Print and shaded views of the part. All mm, measured from the part's lowest x, y and z. A direction names the side the tool comes from. Round coordinates to 2 decimals unless told otherwise and drop trailing zeros. Write each loop counter-clockwise with the first axis right and the second up, starting at its lowest first coordinate (ties: lowest second). Pieces come first, ordered by that corner, then holes. Notation, with made-up numbers: (51, -0.5) - (59, -0.5) arc R13 cw to (59, 6.5) - close; hole circle Ø6 at (-21.75, 88.5). An arc over 180 degrees is marked (long way). Put each result on its own line as item: value. Start each with the question number.
Item 1: 3-axis set-ups, long thin cutter, end or side, ignore diameter. For the marked faces 1, 2 and 3: which of +Z, -Z, +X, -X, +Y, -Y reach the whole face in a straight line?
Item 2: Cut at D-D (x = 40.5). Give the cut face in (y, z), and give its area (3 significant figures).
Item 3: Pin check, flat tips, straight feed: pin 1 Ø0.7 at (y, z) = (9.5, 5) entering from -X; pin 2 Ø0.8 at (y, z) = (1.5, 3) entering from -X; pin 3 Ø1.4 at (y, z) = (0.5, 3) entering from +X. Stop position of each tip, or through.
Item 4: Cut at C-C (z = 5). Give the cut face in (x, y), and give its area (3 significant figures).
Item 5: Drill centre lines: line 1 (Y direction, x = 20, z = 4.75); line 2 (X direction, y = 12.75, z = 4.25); line 3 (X direction, y = 10.75, z = 3.5). Where is each one in solid material? Low to high. Write a range as from..to.
Item 6: Cut at A-A (x = 20). Give the cut face in (y, z), and give its area (3 significant figures).
Item 7: Cut at B-B (y = 11.15). Give the cut face in (x, z) (3 decimals), and give its area (3 significant figures).
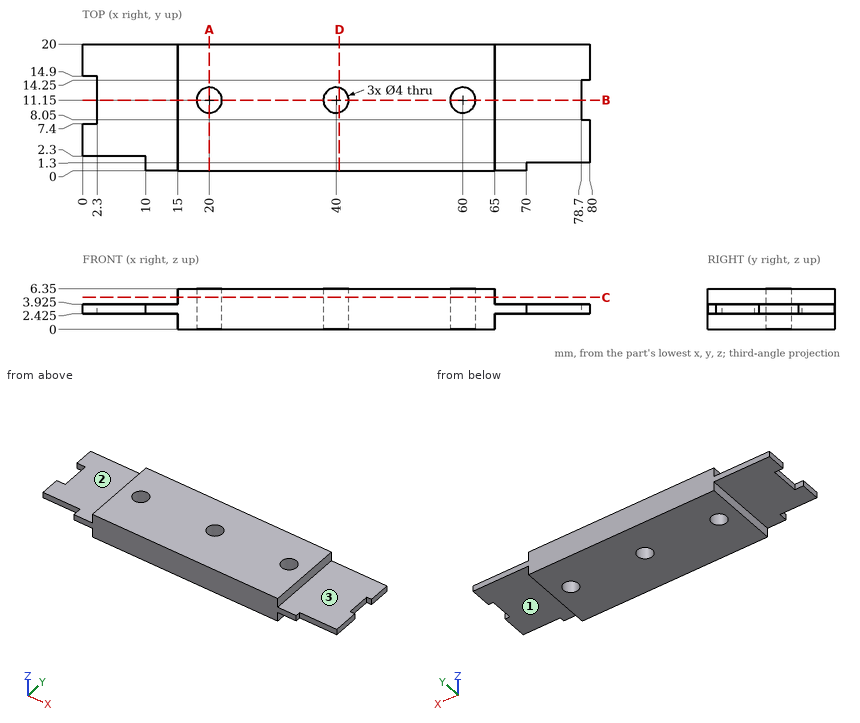
Output values:
1. face 1: -Z, +X, +Y, -Y
1. face 2: +Z, -X, +Y, -Y
1. face 3: +Z, +X, +Y, -Y
2. outline: (0, 0) - (9.21, 0) - (9.21, 6.35) - (0, 6.35) - close; (13.09, 0) - (20, 0) - (20, 6.35) - (13.09, 6.35) - close
2. area: 102 mm2
3. pin 1: x = 15
3. pin 2: x = 10
3. pin 3: x = 70
4. outline: (15, 0) - (65, 0) - (65, 20) - (15, 20) - close; hole circle Ø4 at (20, 11.15); hole circle Ø4 at (40, 11.15); hole circle Ø4 at (60, 11.15)
4. area: 962 mm2
5. line 1: 0..9.15, 13.15..20
5. line 2: 15..18.8, 21.2..38.8, 41.2..58.8, 61.2..65
5. line 3: 2.3..18.04, 21.96..38.04, 41.96..58.04, 61.96..78.7
6. outline: (0, 0) - (9.15, 0) - (9.15, 6.35) - (0, 6.35) - close; (13.15, 0) - (20, 0) - (20, 6.35) - (13.15, 6.35) - close
6. area: 102 mm2
7. outline: (2.3, 2.425) - (15, 2.425) - (15, 0) - (18, 0) - (18, 6.35) - (15, 6.35) - (15, 3.925) - (2.3, 3.925) - close; (22, 0) - (38, 0) - (38, 6.35) - (22, 6.35) - close; (42, 0) - (58, 0) - (58, 6.35) - (42, 6.35) - close; (62, 0) - (65, 0) - (65, 2.425) - (78.7, 2.425) - (78.7, 3.925) - (65, 3.925) - (65, 6.35) - (62, 6.35) - close
7. area: 281 mm2
